from build123d import *

# Parameters (mm, degrees)
SKETCH1_W               = 150
SKETCH1_H               = 125
BOSS_EXTRUDE1_DEPTH     = 37.5
CUT_EXTRUDE1_DEPTH      = 124.110722522
CUT_EXTRUDE1_DEPTH_BACK = 5
SKETCH2_R               = 45
CUT_EXTRUDE2_REACH      = 122.13
SKETCH3_R               = 26
SKETCH4_R               = 26
BOSS_EXTRUDE2_DEPTH     = 16
SKETCH5_R               = 20
BOSS_EXTRUDE3_DEPTH     = 10.5
SKETCH6_R               = 26
BOSS_EXTRUDE4_DEPTH     = 13.5


with BuildPart() as part:
    # Sketch1 → Boss-Extrude1 (new, symmetric)
    with BuildSketch(Plane(origin=(0, 0, 0), x_dir=(0, 1, 0), z_dir=(0, 0, 1))):
        Rectangle(SKETCH1_W, SKETCH1_H)
    extrude(amount=BOSS_EXTRUDE1_DEPTH, both=True)

    # Sketch2 → Cut-Extrude1 (cut, two sides: drawn at the far end of the back side and taken through both)
    with BuildSketch(Plane.XY.offset(37.5).offset(-CUT_EXTRUDE1_DEPTH_BACK)):
        with Locations(Location((0, 0, 0), (0, 0, 180))):
            Circle(SKETCH2_R)
    extrude(amount=CUT_EXTRUDE1_DEPTH + CUT_EXTRUDE1_DEPTH_BACK, mode=Mode.SUBTRACT)

    # Sketch3 → Cut-Extrude2 (cut, up to next)
    with BuildSketch(Plane.XY.offset(32.5), mode=Mode.PRIVATE) as cut_extrude2_sk1:
        Circle(SKETCH3_R)
    cut_extrude2_tool1 = extrude(cut_extrude2_sk1.sketch, amount=-CUT_EXTRUDE2_REACH, mode=Mode.PRIVATE) & part.part
    add(cut_extrude2_tool1.solids().sort_by_distance((0, 0, 32.5))[0], mode=Mode.SUBTRACT)

    # Sketch4 → Boss-Extrude2 (add)
    with BuildSketch(Plane(origin=(0, 75, 0), x_dir=(-1, 0, 0), z_dir=(0, 1, 0))):
        Circle(SKETCH4_R)
    boss_extrude2 = extrude(amount=BOSS_EXTRUDE2_DEPTH)

    # Sketch5 → Boss-Extrude3 (add)
    with BuildSketch(Plane(origin=(0, 91, 0), x_dir=(-1, 0, 0), z_dir=(0, 1, 0))):
        with Locations(Location((0, 0, 0), (0, 0, 180))):
            Circle(SKETCH5_R)
    boss_extrude3 = extrude(amount=BOSS_EXTRUDE3_DEPTH)

    # Sketch6 → Boss-Extrude4 (add)
    with BuildSketch(Plane(origin=(0, 101.5, 0), x_dir=(-1, 0, 0), z_dir=(0, 1, 0))):
        Circle(SKETCH6_R)
    boss_extrude4 = extrude(amount=BOSS_EXTRUDE4_DEPTH)

    # Mirror1: Boss-Extrude2, Boss-Extrude3, Boss-Extrude4 across plane
    add(boss_extrude2.mirror(Plane.ZX))
    add(boss_extrude3.mirror(Plane.ZX))
    add(boss_extrude4.mirror(Plane.ZX))


solid = part.part
Could you check a few things on this model? Use its own coordinates, in mm. A direction names the side the tool comes from. Give positions to 0.01 mm unless a question says otherwise; leave off trailing zeros. Order: outer loops, then holes, each group sorted by start corner. A loop starts at its lowest first (then second) coordinate and runs counter-clockwise, first axis right, second up. Notation, with made-up numbers: (-23.75, 74.25) - (9.25, 74.25) arc R13 ccw to (9.25, 84.25) - close; hole circle Ø7 at (-38, -3). An arc over 180 degrees is marked (long way). Return JSON: item names as keys, results as strings. Group by question number.
Q1. Suppose I cut it at D-D, the plane z = 23.5. Please give me the cut outline in (x, y).
Q2. Suppose I cut it at C-C, the plane x = 23. Please give me the cut outline in (y, z).
Q3. Will these pins go through, and if not, where does the flat tip stop? pin 1 Ø8 at (y, z) = (-84.5, 14.5) entering from -X; pin 2 Ø2 at (x, y) = (-2.5, 76.5) entering from +Z; pin 3 Ø2 at (x, z) = (32.5, -26) entering from -Y.
Q4. Please list where these lines run through material, in increasing order: line 1 along Y through (x, z) = (0, 36); line 2 along Y through (x, z) = (-17, -16); line 3 along Y through (x, z) = (0, 17). Write a range as [from, to].
Q5. Suppose I cut it at A-A, the plane y = 0. Please give me the cut outline in (x, z), and give its area (4 significant figures).
Q6. Which directions (+Z, -Z, +X, -X, +Y, -Y) give clear straight access to the entire face, cutting with the end or side of a thin tool? Please do faces 1 (the face through (20.633, 82.888, -15.821)), 2 (the face through (20.633, -82.888, -15.821)), 3 (the face through (-13.4, 101.5, -15.3)), 4 (the face through (-20.765, 39.923, 34.965)).
Q7. Thinking about a two-plate mould opening in X: for faces 5 (the face through (20.633, -108.156, -15.821)), 6 (the face through (0, -115, 0)), 7 (the face through (-19, 19, 32.5)), 8 (the face through (62.5, -1, 1)), which applies, pulls with the +X half, pulls with the -X half, needs draft (parallel to the pull), parting line crosses it, or undercut?
Resolved:
{
 "1": {"outline": "(-62.5, -75) - (-11.12, -75) - (-11.12, -91) - (11.12, -91) - (11.12, -75) - (62.5, -75) - (62.5, 75) - (11.12, 75) - (11.12, 91) - (-11.12, 91) - (-11.12, 75) - (-62.5, 75) - close; (-11.12, -115) - (11.12, -115) - (11.12, -101.5) - (-11.12, -101.5) - close; (-11.12, 101.5) - (11.12, 101.5) - (11.12, 115) - (-11.12, 115) - close; hole circle Ø52 at (0, 0)"},
 "2": {"outline": "(-115, -12.12) - (-101.5, -12.12) - (-101.5, 12.12) - (-115, 12.12) - close; (-91, -12.12) - (-75, -12.12) - (-75, -37.5) - (-12.12, -37.5) - (-12.12, 32.5) - (-38.68, 32.5) - (-38.68, 37.5) - (-75, 37.5) - (-75, 12.12) - (-91, 12.12) - close; (12.12, -37.5) - (75, -37.5) - (75, -12.12) - (91, -12.12) - (91, 12.12) - (75, 12.12) - (75, 37.5) - (38.68, 37.5) - (38.68, 32.5) - (12.12, 32.5) - close; (101.5, -12.12) - (115, -12.12) - (115, 12.12) - (101.5, 12.12) - close"},
 "3": {"pin 1": "stops at x = -23.79", "pin 2": "stops at z = 25.96", "pin 3": "stops at y = -75"},
 "4": {"line 1": "y = [-75, -45], [45, 75]", "line 2": "y = [-115, -101.5], [-91, -19.67], [19.67, 91], [101.5, 115]", "line 3": "y = [-115, -26], [26, 115]"},
 "5": {"outline": "(-62.5, -37.5) - (-26, -37.5) - (-26, 32.5) - (-45, 32.5) - (-45, 37.5) - (-62.5, 37.5) - close; (26, -37.5) - (62.5, -37.5) - (62.5, 37.5) - (45, 37.5) - (45, 32.5) - (26, 32.5) - close", "area": "5,285 mm2"},
 "6": {"face 1": "+Y", "face 2": "-Y", "face 3": "none", "face 4": "+Z"},
 "7": {"face 5": "parting line crosses it", "face 6": "needs draft", "face 7": "undercut", "face 8": "pulls with the +X half"}
}
